Geometry: see drawing. Coordinates: mm, zero at the bounding-box minimum. Give positions to 0.01 mm unless a question says otherwise; leave off trailing zeros. Write each loop counter-clockwise with the first axis right and the second up, starting at its lowest first coordinate (ties: lowest second). Pieces come first, ordered by that corner, then holes. Notation, with made-up numbers: (-21.75, 42.25) -> (-16.75, 42.25) arc R31 cw to (-16.75, 75.25) -> close; hole circle Ø10 at (31.25, 24). An arc over 180 degrees is marked (long way). Answer as a JSON object with one key per item and string values. Group by question number.
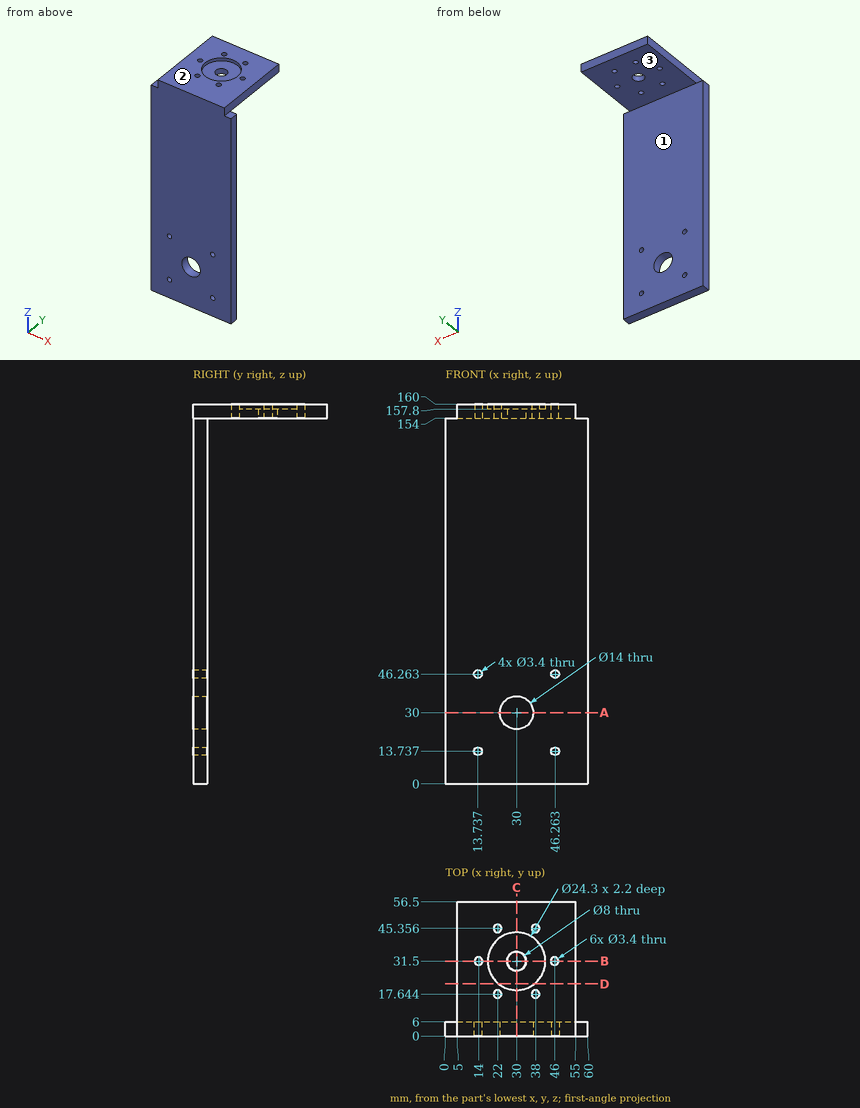
1. Line query: line 1 (Y direction, x = 38, z = 156.7); line 2 (Y direction, x = 46, z = 157.65); line 3 (Y direction, x = 30, z = 155.3). Output: solid intervals per line, ascending.
2. Section C-C (x = 30). Return the cut outline in (y, z).
3. Section D-D (y = 22). Return the cut outline in (x, z) (1 decimal), plus the area to 3 significant figures.
4. Contact query for flat-ended pins moving along their axis: pin 1 Ø22 at (x, y) = (30, 31.5) entering from +Z; pin 2 Ø3 at (y, z) = (39.5, 157.5) entering from -X; pin 3 Ø18 at (x, z) = (24.5, 77) entering from +Y; pin 4 Ø6.5 at (x, y) = (30, 31.5) entering from -Z. Output: stop coordinate, or through.
5. Section B-B (y = 31.5). Return the cut outline in (x, z).
6. Mould query, pull axis Z, two halves, no side actions, for the marked faces 1, 2 and 3. Classes: pulls with the +Z half, pulls with the -Z half, needs draft (parallel to the pull), parting line crosses it, or undercut.
7. Section A-A (z = 30). Return the cut outline in (x, y), plus the area to 3 significant figures.
Working result:
{
 "1": {"line 1": "y = 0 to 15.94, 19.34 to 43.66, 47.06 to 56.5", "line 2": "y = 0 to 29.8, 33.2 to 56.5", "line 3": "y = 0 to 27.5, 35.5 to 56.5"},
 "2": {"outline": "(0, 0) -> (6, 0) -> (6, 23) -> (0, 23) -> close; (0, 37) -> (6, 37) -> (6, 154) -> (27.5, 154) -> (27.5, 157.8) -> (19.35, 157.8) -> (19.35, 160) -> (0, 160) -> close; (35.5, 154) -> (56.5, 154) -> (56.5, 160) -> (43.65, 160) -> (43.65, 157.8) -> (35.5, 157.8) -> close"},
 "3": {"outline": "(5, 154) -> (55, 154) -> (55, 160) -> (37.6, 160) -> (37.6, 157.8) -> (22.4, 157.8) -> (22.4, 160) -> (5, 160) -> close", "area": "267 mm^2"},
 "4": {"pin 1": "stops at z = 157.8", "pin 2": "stops at x = 5", "pin 3": "stops at y = 6", "pin 4": "passes through"},
 "5": {"outline": "(5, 154) -> (12.3, 154) -> (12.3, 160) -> (5, 160) -> close; (15.7, 154) -> (26, 154) -> (26, 157.8) -> (17.85, 157.8) -> (17.85, 160) -> (15.7, 160) -> close; (34, 154) -> (44.3, 154) -> (44.3, 160) -> (42.15, 160) -> (42.15, 157.8) -> (34, 157.8) -> close; (47.7, 154) -> (55, 154) -> (55, 160) -> (47.7, 160) -> close"},
 "6": {"face 1": "needs draft", "face 2": "pulls with the +Z half", "face 3": "pulls with the -Z half"},
 "7": {"outline": "(0, 0) -> (23, 0) -> (23, 6) -> (0, 6) -> close; (37, 0) -> (60, 0) -> (60, 6) -> (37, 6) -> close", "area": "276 mm^2"}
}
